Work out the finished part from the listing and answer in its coordinate system (mm). A direction names the side the tool comes from. Give positions to 0.01 mm unless a question says otherwise; leave off trailing zeros. Write each loop counter-clockwise with the first axis right and the second up, starting at its lowest first coordinate (ties: lowest second). Pieces come first, ordered by that corner, then holes. Notation, with made-up numbers: (88.5, 37.25) - (107.5, 37.25) arc R24 cw to (107.5, 72.25) - close; hole circle Ø6 at (2.5, 68). An arc over 180 degrees is marked (long way). Write each question's results on one line, items separated by ' | '. Start each with the question number.
from build123d import *

# Parameters (mm, degrees)
BOSS_EXTRUDE1_DEPTH      = 50.8
BOSS_EXTRUDE1_DEPTH_BACK = 50.8
SKETCH1_W                = 1.524
SKETCH1_H                = 4.871067054
CUT_EXTRUDE1_DEPTH       = 50.8
CUT_EXTRUDE1_DEPTH_BACK  = 50.8
SKETCH2_OUTSIDE_W        = 135.154
SKETCH2_OUTSIDE_H        = 148.693


with BuildPart() as part:
    # Sketch1 → Boss-Extrude1 (new, two sides: drawn at the far end of the back side and taken through both)
    with BuildSketch(Plane.XY.offset(-BOSS_EXTRUDE1_DEPTH_BACK)):
        with BuildLine():
            ThreePointArc((6.741617203, 20.144109787), (1.698900198, 22.631956132), (-3.343816807, 20.144109787))
            ThreePointArc((-3.343816807, 20.144109787), (-5.71730664, 13.971140244), (-7.597975628, 7.630628347))
            ThreePointArc((-7.597975628, 7.630628347), (-8.701431417, -34.535652594), (-3.014754354, -76.331281159))
            ThreePointArc((-3.014754354, -76.331281159), (1.525815948, -85.900303593), (9.804659046, -92.506643425))
            ThreePointArc((9.804659046, -92.506643425), (19.466075818, -86.644924226), (24.084678714, -76.331281159))
            ThreePointArc((24.084678714, -76.331281159), (25.152625845, -26.342752003), (6.741617203, 20.144109787))
        make_face()
        with Locations((-0.762, 13.555168851)):
            Rectangle(SKETCH1_W, SKETCH1_H, mode=Mode.SUBTRACT)
    extrude(amount=BOSS_EXTRUDE1_DEPTH + BOSS_EXTRUDE1_DEPTH_BACK)

    # Sketch2 outside → Cut-Extrude1 (cut, two sides: drawn at the far end of the back side and taken through both)
    with BuildSketch(Plane(origin=(0, 0, 0), x_dir=(0, 0, -1), z_dir=(1, 0, 0)).offset(-CUT_EXTRUDE1_DEPTH_BACK)):
        with Locations((0, -34.9375)):
            Rectangle(SKETCH2_OUTSIDE_W, SKETCH2_OUTSIDE_H)
        with BuildLine():
            Line((1.509494799, 22.422190899), (0, 22.631956132))
            ThreePointArc((0, 22.631956132), (-3.980899399, -34.937343647), (0, -92.506643425))
            Line((0, -92.506643425), (1.509494799, -92.296878192))
            ThreePointArc((1.509494799, -92.296878192), (-2.456899399, -34.937343647), (1.509494799, 22.422190899))
        make_face(mode=Mode.SUBTRACT)
    extrude(amount=CUT_EXTRUDE1_DEPTH + CUT_EXTRUDE1_DEPTH_BACK, mode=Mode.SUBTRACT)


solid = part.part
Q1. A tool of negligible diameter and unlimited length cuts with its end or side. For faces 1 (the cylindrical face through (-1.643, 21.682, -0.599)), 2 (the flat face through (-1.524, 14, 0)), from which of +Z, -Z, +X, -X, +Y, -Y can it reach the whole face along a straight path? Write none if from no direction.
Q2. The mould has two halves that part along X. Classify faces 3 (the cylindrical face through (-5.687, 14.059, 0.284)), 4 (the flat face through (0, 14, 0)), 5 (the cylindrical face through (19.359, -86.765, 0.185)): pulls with the +X half, pulls with the -X half, needs draft (parallel to the pull), parting line crosses it, or undercut.
Q3. A cutting plane is placed at C-C, the plane y = -16. Write down the section's boundary in (x, z).
Q4. Given pin 1 (0.8 mm diameter, centred on x = -1, z = 0, fed in from -Y); pin 2 (1.5 mm diameter, centred on x = 7, y = -56, fed in from -Z); pin 3 (2 mm diameter, centred on x = 16, z = 0.5, fed in from -Y), each flat-ended and moving along its own axis, determine where each tip first touches the part or whether it passes through.
Q5. A cutting plane is placed at A-A, the plane y = 14.5. Write down the section's boundary in (x, z), and give its area (3 significant figures).
Q6. A cutting plane is placed at B-B, the plane x = 16. Write down the section's boundary in (y, z), and give its area (3 significant figures).
Q7. Consider L1, parallel to X at y = -48, z = 3.3; L2, parallel to X at y = -70, z = 1.4; L3, parallel to Z at x = 3, y = -17.5. Determine where each line is inside the solid, lowest interval first.
Result:
1) face 1: +Z, -Z, -X, +Y | face 2: +Z, -Z
2) face 3: pulls with the -X half | face 4: undercut | face 5: pulls with the +X half
3) outline: (-9.06, 2.03) - (22.84, 2.03) - (22.84, 3.55) - (-9.06, 3.55) - close
4) pin 1: stops at y = -82.72 | pin 2: stops at z = 1.89 | pin 3: stops at y = -90.35
5) outline: (-5.54, -0.49) - (-1.52, -0.49) - (-1.52, 1.05) - (-5.54, 1.05) - close; (0, -0.49) - (10.2, -0.49) - (10.2, 1.05) - (0, 1.05) - close | area: 21.8 mm2
6) outline: (-89.72, -1.16) arc R416.73 cw to (3.19, 0.71) - (3.19, 2.24) arc R418.26 ccw to (-89.72, 0.38) - close | area: 142 mm2
7) L1: x = -7.62 to 27.14 | L2: x = -4.32 to 25.34 | L3: z = 2.09 to 3.62
